from build123d import *

# Parameters (mm, degrees)
F0_R     = 22
F0_R_2   = 19
F1_DEPTH = 7
F2_SIZE  = 1.5
F3_R     = 22
F3_R_2   = 19
F4_DEPTH = 3
F5_SIZE  = 1.49999
F6_SIZE  = 2.5
F7_SIZE  = 1.5
F8_R     = 22
F8_R_2   = 19
F9_DEPTH = 2
F10_SIZE = 1.49999


# Not quite as in the source:
# - a fillet or chamfer is up to 0.001 mm smaller than in the source, because OpenCascade refuses the exact size


with BuildPart() as f1:
    # F0 (on Front) → F1 (new body)
    with BuildSketch(Plane.XZ):
        Circle(F0_R)
        Circle(F0_R_2, mode=Mode.SUBTRACT)
    extrude(amount=F1_DEPTH)

    # F2
    f2_edges = [f1.edges().sort_by_distance(p)[0] for p in [
        (-22, 0, 0),
    ]]
    chamfer(f2_edges, length=F2_SIZE)

    # F3 (on face) → F4 (join)
    with BuildSketch(Plane(origin=(0, 0, 0), x_dir=(-1, 0, 0), z_dir=(0, 1, 0))):
        Circle(F3_R)
        Circle(F3_R_2, mode=Mode.SUBTRACT)
    extrude(amount=F4_DEPTH)

    # F5 (size 1.5 in the source; OpenCascade refuses exactly that, so slightly less here)
    f5_edges = [f1.edges().sort_by_distance(p)[0] for p in [
        (22, 0, 0),
    ]]
    chamfer(f5_edges, length=F5_SIZE)

    # F6
    f6_edges = [f1.edges().sort_by_distance(p)[0] for p in [
        (19, 3, 0),
    ]]
    chamfer(f6_edges, length=F6_SIZE)

    # F7
    f7_edges = [f1.edges().sort_by_distance(p)[0] for p in [
        (-22, -7, 0),
    ]]
    chamfer(f7_edges, length=F7_SIZE)

    # F8 (on face) → F9 (join)
    with BuildSketch(Plane.XZ.offset(7)):
        Circle(F8_R)
        Circle(F8_R_2, mode=Mode.SUBTRACT)
    extrude(amount=F9_DEPTH)

    # F10 (size 1.5 in the source; OpenCascade refuses exactly that, so slightly less here)
    f10_edges = [f1.edges().sort_by_distance(p)[0] for p in [
        (-22, -7, 0),
    ]]
    chamfer(f10_edges, length=F10_SIZE)


solid = f1.part
Input: part model. Units: mm. Frame: model coordinates. Give positions to 0.01 mm unless a question says otherwise; leave off trailing zeros. Order: outer loops, then holes, each group sorted by start corner. A loop starts at its lowest first (then second) coordinate and runs counter-clockwise, first axis right, second up.
Q1. Contact query for flat-ended pins moving along their axis: pin 1 Ø3 at (x, y) = (-8.5, -6) entering from -Z; pin 2 Ø1.5 at (y, z) = (1.5, 11) entering from +X; pin 3 Ø2 at (x, y) = (4.5, -6) entering from -Z. Output: stop coordinate, or through.
Checked values:
pin 1: stops at z = -20.83
pin 2: stops at x = 19.47
pin 3: stops at z = -21.7
Q2. Draft query along X for faces 1 (the cylindrical face through (4.769, 2.239, -21.477)), 2 (the conical face through (4.145, 0.621, -18.667)), 3 (the flat face through (-9.7, 3, -19.5)). Return one class per face: +X half, -X half, draft (parallel to the pull), parting line (faces both ways), or undercut.
Checked values:
face 1: parting line
face 2: undercut
face 3: draft
Q3. Section C-C on y = -2.5. Output: boundary loops of the cut face in (x, z).
Checked values:
outline: circle Ø44 at (0, 0); hole circle Ø38 at (0, 0)
Q4. Ray query, probe 1 along Z at (x, y) = (0, -2.5); probe 2 along Z at (x, y) = (0, -7.45); probe 3 along X at (y, z) = (-1, 11). Return the intervals inside material, ascending.
Checked values:
probe 1: z = -22 to -19, 19 to 22
probe 2: z = -20.95 to -19, 19 to 20.95
probe 3: x = -18.47 to -15.49, 15.49 to 18.47
